Design review of the part built by this model. Coordinates are the model's own, in mm. A direction names the side the tool comes from. Coordinates: 2 decimals unless noted, no trailing zeros. Write each loop counter-clockwise with the first axis right and the second up, starting at its lowest first coordinate (ties: lowest second). Pieces come first, ordered by that corner, then holes. Notation, with made-up numbers: (4, 88.25) -> (17, 88.25) arc R23 ccw to (17, 98.25) -> close; hole circle Ø5 at (8, 32.5). An arc over 180 degrees is marked (long way). Write item = value, one per line. Start each with the question number.
```python
from build123d import *

# Parameters (mm, degrees)
F1_DEPTH = 23
F2_W     = 113
F2_H     = 46
F3_DEPTH = 40
F4_R     = 7
F5_R     = 10
F6_W     = 113
F6_H     = 6
F7_DEPTH = 200.001


with BuildPart() as f1:
    # F0 (on Front) → F1 (new body, symmetric)
    with BuildSketch(Plane.XZ):
        Polygon((0, 160), (0, 0), (74, 0), (74, 125), (113, 125), (113, 160), align=None)
    extrude(amount=F1_DEPTH, both=True)

    # F2 (on face) → F3 (join)
    with BuildSketch(Plane.XY.offset(160)):
        with Locations((56.5, 0)):
            Rectangle(F2_W, F2_H)
    extrude(amount=F3_DEPTH)

    # F4
    f4_edges = [f1.edges().sort_by_distance(p)[0] for p in [
        (74, 0, 0),
        (0, 0, 0),
        (113, 0, 125),
    ]]
    fillet(f4_edges, radius=F4_R)

    # F5
    f5_edges = [f1.edges().sort_by_distance(p)[0] for p in [
        (74, 0, 125),
    ]]
    fillet(f5_edges, radius=F5_R)

    # F6 (on face) → F7 (cut, through all)
    with BuildSketch(Plane.XY.offset(200)):
        with Locations((56.5, 20)):
            Rectangle(F6_W, F6_H)
    extrude(amount=-F7_DEPTH, mode=Mode.SUBTRACT)


solid = f1.part
```
(1) Take a section at B-B, the plane z = 96. State the section outline as (x, y) points.
(2) For line 1 (X direction, y = 13.5, z = 59); line 2 (Z direction, x = 104.5, y = -12); line 3 (Z direction, x = 78, y = -16.5), list the stretches that pass through material, from the lowest coordinate up.
(3) For pin 1 Ø5 at (x, y) = (73, -5) entering from -Z; pin 2 Ø10 at (y, z) = (-17.5, 95) entering from +X; pin 3 Ø1 at (x, y) = (70.5, 6) entering from -Z, all flat-tipped, find the tip position at first contact; note any pin that passes through.
(4) Take a section at C-C, the plane x = 95. State the section outline as (y, z) points.
(5) For faces 1 (the face through (74, -3, 60)), 2 (the face through (56, -3, 200)), list the 3-axis set-ups (+Z, -Z, +X, -X, +Y, -Y) from which the entire face can be reached by the end or side of a thin tool; tool diameter is ignored.
(6) Take a section at A-A, the plane y = -12. State the section outline as (x, z) points, then the cut area to 3 significant figures.
Report:
q1.outline = (0, -23) -> (74, -23) -> (74, 17) -> (0, 17) -> close
q2.line_1 = 0 to 74
q2.line_2 = 125 to 200
q2.line_3 = 123 to 200
q3.pin_1 = 0.94
q3.pin_2 = 74
q3.pin_3 = 0.68
q4.outline = (-23, 125) -> (17, 125) -> (17, 200) -> (-23, 200) -> close
q5.face_1 = -Z, +X, +Y, -Y
q5.face_2 = +Z, +X, -X, +Y, -Y
q6.outline = (0, 7) arc R7 ccw to (7, 0) -> (67, 0) arc R7 ccw to (74, 7) -> (74, 115) arc R10 cw to (84, 125) -> (106, 125) arc R7 ccw to (113, 132) -> (113, 200) -> (0, 200) -> close
q6.area = 17,700 mm2
